The listing builds one solid part. Answer for the finished solid, in the listing's coordinates (mm). A direction names the side the tool comes from. Coordinates: 2 decimals unless noted, no trailing zeros. Put each result on its own line as item: value.
Autodesk Inventor part; units mm, degrees
ref_plane "YZ Plane" through (0, 0, 0) normal (1, 0, 0) x (0, 1, 0)
ref_plane "XZ Plane" through (0, 0, 0) normal (0, 1, 0) x (-1, 0, 0)
ref_plane "XY Plane" through (0, 0, 0) normal (0, 0, 1) x (1, 0, 0)
sketch "Sketch2" plane through (0, 0, 0) normal (0, 0, 1) x (1, 0, 0)
  arc A0 (-28.6864, 13.6071) -> (28.6864, 13.6071) centre (0, 0) ccw
  arc A1 (11.4746, 49.8929) -> (-11.4746, 49.8929) centre (0, 44.45) ccw
  line L0 (-28.6864, 13.6071) -> (-11.4746, 49.8929)
  line L1 (11.4746, 49.8929) -> (28.6864, 13.6071)
  line L2 (-1.5875, -1.5875) -> (-1.5875, 1.5875)
  line L3 (-1.5875, 1.5875) -> (1.5875, 1.5875)
  line L4 (1.5875, 1.5875) -> (1.5875, -1.5875)
  line L5 (1.5875, -1.5875) -> (-1.5875, -1.5875)
  line L6 (-1.5875, -1.5875) -> (1.5875, 1.5875) construction
  line L7 (-1.5875, 1.5875) -> (1.5875, -1.5875) construction
  dimension "d16" = 63.5
  dimension "d18" = 25.4
  dimension "d19" = 44.45
  dimension "d22" = 3.175
  dimension "d23" = 3.175
extrude "Extrusion3" add sketch "Sketch2" along normal blind 3.175
fillet "Fillet3" radius 1.016 8 edges at (0, 57.15, 3.175) (-20.0805, 31.75, 3.175) (0, -31.75, 3.175) (20.0805, 31.75, 3.175) (0, 57.15, 0) (-20.0805, 31.75, 0) (0, -31.75, 0) (20.0805, 31.75, 0)
chamfer "Chamfer1" distance 0.254 angle 45 8 edges at (1.5875, 0, 3.175) (0, -1.5875, 3.175) (-1.5875, 0, 3.175) (0, 1.5875, 3.175) (0, -1.5875, 0) (-1.5875, 0, 0) (0, 1.5875, 0) (1.5875, 0, 0)
properties part number "4.2 Part D"
1) Straight lines are drawn through the part: L1, parallel to Y at x = 1, z = 3.05; L2, parallel to Y at x = -23.5, z = 0.95; L3, parallel to X at y = -5, z = 1.65. For each, find the intervals that lie inside material, in ascending order. Write a range as [from, to].
Found:
L1: y = [-31.21, -1.72], [1.72, 56.58]
L2: y = [-21.35, 24.54]
L3: x = [-31.35, 31.35]
2) For faces 5 (the face through (0, 1.588, 2)), 6 (the face through (0, 13, 0)), determine the directions among +Z, -Z, +X, -X, +Y, -Y from which every point of the face is accessible in a straight line to the end or side of a thin tool.
Found:
face 5: +Z, -Z
face 6: -Z, +X, -X, +Y, -Y
3) Each of these flat-tipped pins is pushed along its axis until it touches: pin 1 (1 mm diameter, centred on x = -8.5, z = 0.5, fed in from -Y); pin 2 (8 mm diameter, centred on x = -10, y = -8, fed in from -Z); pin 3 (0.8 mm diameter, centred on y = 0.5, z = 1, fed in from -X). Where does it stop, or does it pass through?
Found:
pin 1: stops at y = -30.68
pin 2: stops at z = 0
pin 3: stops at x = -31.75
4) For a pull along X with two mould halves and no side action, classify faces 1 (the face through (1.588, 0, 2)), 2 (the face through (19.7, 31.88, 0.31)), 3 (the face through (-19.939, 31.372, 0.306)), 4 (the face through (-1.588, 0, 2)) as pulls with the +X half, pulls with the -X half, needs draft (parallel to the pull), parting line crosses it, or undercut.
Found:
face 1: undercut
face 2: pulls with the +X half
face 3: pulls with the -X half
face 4: undercut
